For this review, take the finished solid that the model builds, in its own axes (mm). A direction names the side the tool comes from. Give positions to 0.01 mm unless a question says otherwise; leave off trailing zeros. Write each loop counter-clockwise with the first axis right and the second up, starting at its lowest first coordinate (ties: lowest second). Pieces come first, ordered by that corner, then holes. Notation, with made-up numbers: (-27, -35.5) -> (28, -35.5) arc R18 cw to (28, -22.5) -> close; hole circle Ø2 at (19.25, 83). An arc over 180 degrees is marked (long way). Write item = value, one per line.
```python
from build123d import *

# Parameters (mm, degrees)
F1_DEPTH = 20
F2_R     = 1.4
F3_W     = 10.1
F3_H     = 2.1
F4_DEPTH = 15
F5_SIZE  = 3
F7_D     = 2.2
F8_D     = 2.7
F9_D     = 3.2
F10_D    = 3.7


with BuildPart() as f1:
    # F0 (on Top) → F1 (new body)
    with BuildSketch(Plane.XY):
        Polygon((-46, -50), (-40, -50), (-34, -50), (-30, -43), (-26, -50), (-20, -50), (-14, -50), (-10, -43), (-6, -50), (0, -50), (6, -50), (10, -43), (14, -50), (20, -50), (26, -50), (30, -43), (34, -50), (40, -50), (46, -50), (50, -43), (54, -50), (60, -50), (60, 50), (-60, 50), (-60, -50), (-54, -50), (-50, -43), align=None)
    extrude(amount=F1_DEPTH)

    # F2
    f2_edges = [f1.edges().sort_by_distance(p)[0] for p in [
        (-50, -43, 10),
        (-30, -43, 10),
        (-10, -43, 10),
        (10, -43, 10),
        (30, -43, 10),
        (50, -43, 10),
    ]]
    fillet(f2_edges, radius=F2_R)

    # F3 (on face) → F4 (cut)
    with BuildSketch(Plane(origin=(0, 0, 0), x_dir=(1, 0, 0), z_dir=(0, 0, -1))):
        with Locations((-49.95, 42.45)):
            Rectangle(F3_W, F3_H)
        with Locations((-29.95, 42.45)):
            Rectangle(F3_W, F3_H)
        with Locations((-9.95, 42.45)):
            Rectangle(F3_W, F3_H)
        with Locations((10.05, 42.45)):
            Rectangle(F3_W, F3_H)
        with Locations((30.05, 42.45)):
            Rectangle(F3_W, F3_H)
        with Locations((50.05, 42.45)):
            Rectangle(F3_W, F3_H)
    extrude(amount=-F4_DEPTH, mode=Mode.SUBTRACT)

    # F5
    f5_edges = [f1.edges().sort_by_distance(p)[0] for p in [
        (0, 50, 20),
        (-40, -50, 20),
        (-57, -50, 20),
        (-20, -50, 20),
        (0, -50, 20),
        (20, -50, 20),
        (40, -50, 20),
        (57, -50, 20),
    ]]
    chamfer(f5_edges, length=F5_SIZE)

    # F7 (through all)
    with Locations(Plane.XY.offset(20)):
        with Locations((50, -25), (30, -25)):
            Hole(F7_D / 2)

    # F8 (through all)
    with Locations(Plane.XY.offset(20)):
        with Locations((50, 10), (30, 10), (10, 10), (10, -25)):
            Hole(F8_D / 2)

    # F9 (through all)
    with Locations(Plane.XY.offset(20)):
        with Locations((-10, 10), (-30, 10), (-10, -25)):
            Hole(F9_D / 2)

    # F10 (through all)
    with Locations(Plane.XY.offset(20)):
        with Locations((-50, 10)):
            Hole(F10_D / 2)


solid = f1.part
```
(1) For pin 1 (1 mm diameter, centred on x = 31, y = -42, fed in from -Z); pin 2 (3 mm diameter, centred on x = 12, z = 16.5, fed in from -Y) (3 decimals); pin 3 (2 mm diameter, centred on x = 10, y = 10, fed in from -Z), all flat-tipped, find the tip position at first contact; note any pin that passes through.
Answers below:
pin_1 = 15
pin_2 = -49.125
pin_3 = through
(2) Take a section at A-A (y = 10). Write out the cut boundary in (x, z).
Answers below:
outline = (-60, 0) -> (-51.85, 0) -> (-51.85, 20) -> (-60, 20) -> close; (-48.15, 0) -> (-31.6, 0) -> (-31.6, 20) -> (-48.15, 20) -> close; (-28.4, 0) -> (-11.6, 0) -> (-11.6, 20) -> (-28.4, 20) -> close; (-8.4, 0) -> (8.65, 0) -> (8.65, 20) -> (-8.4, 20) -> close; (11.35, 0) -> (28.65, 0) -> (28.65, 20) -> (11.35, 20) -> close; (31.35, 0) -> (48.65, 0) -> (48.65, 20) -> (31.35, 20) -> close; (51.35, 0) -> (60, 0) -> (60, 20) -> (51.35, 20) -> close
(3) Take a section at B-B (z = 10.5). Count the separate pieces of the cut face and the enclosed holes in it, plus the area to 3 significant figures.
Answers below:
separate_pieces = 1
enclosed_holes = 16
area = 11,600 mm^2
(4) To check wall thickness, follow probe 1 along Y at (x, z) = (50, 14); probe 2 along Y at (x, z) = (-30, 12); probe 3 along Y at (x, z) = (-10, 5.5). State the ranges of each line that lie inside material, in increasing order.
Answers below:
probe_1 = -44.42 to -43.5, -41.4 to -26.1, -23.9 to 8.65, 11.35 to 50
probe_2 = -44.42 to -43.5, -41.4 to 8.4, 11.6 to 50
probe_3 = -44.42 to -43.5, -41.4 to -26.6, -23.4 to 8.4, 11.6 to 50
(5) The part is to be moulded in two halves that separate along Y. For faces 1 (the face through (27.37, -47.6, 9.86)), 2 (the face through (1, 49, 18)), 3 (the face through (-10, -43.5, 7)), 4 (the face through (-1, 1, 0)), say which applies: released by +Y, released by -Y, zero draft, split by the parting line, or undercut.
Answers below:
face_1 = released by -Y
face_2 = released by +Y
face_3 = undercut
face_4 = zero draft
(6) Tool access review of faces 5 (the face through (30, -43.5, 7)), 6 (the face through (7.37, -47.6, 9.86)), 7 (the face through (-48.532, 8.874, 9.86)): name each direction out of +Z, -Z, +X, -X, +Y, -Y from which nothing blocks a thin tool from reaching the whole face with its end or side.
Answers below:
face_5 = -Z
face_6 = +Z, -Z, -Y
face_7 = +Z, -Z
